Read the model definition and answer for the solid it produces. Units are mm, in the model's axes. A direction names the side the tool comes from. Give positions to 0.01 mm unless a question says otherwise; leave off trailing zeros. Write each loop counter-clockwise with the first axis right and the second up, starting at its lowest first coordinate (ties: lowest second). Pieces come first, ordered by that corner, then holes. Notation, with made-up numbers: M 77,-25.75 L 120,-25.75 A21 ccw 120,-4.75 Z; hole C 6,-2.5 d6. An arc over 180 degrees is marked long. Use a Markdown table: item, result. Add a question column.
Item 1: A cutting plane is placed at C-C on z = -16. Determine the outline of the cut face in (x, y), then the cut area to 3 significant figures.
Item 2: A cutting plane is placed at B-B on y = -10. Determine the outline of the cut face in (x, z), then the cut area to 3 significant figures.
Item 3: Given P1, Ø10, axis at x = 15, z = 5, coming from the +Y side; P2, Ø5, axis at x = 5, z = -15.5, coming from the -Y side; P3, Ø5, axis at x = -10.5, y = -17, coming from the -Z side, each flat-ended and moving along its own axis, determine where each tip first touches the part or whether it passes through.
Item 4: A cutting plane is placed at A-A on x = 0. Determine the outline of the cut face in (y, z), then the cut area to 3 significant figures.
Item 5: The mould has two halves that part along X. Classify faces 1 (the flat face through (25.588, -25, 0)), 2 (the cylindrical face through (-19.523, -50.493, 0.282)), 3 (the flat face through (-13, -51, 0)), 4 (the flat face through (-24.412, -25, 0)): pulls with the +X half, pulls with the -X half, needs draft (parallel to the pull), parting line crosses it, or undercut.
Item 6: For faces 5 (the flat face through (0, -25, 25.086)), 6 (the cylindrical face through (-0.98, -33.78, -25.41)), 7 (the flat face through (0, -50, 0)), determine the directions among +Z, -Z, +X, -X, +Y, -Y from which every point of the face is accessible in a straight line to the end or side of a thin tool.
Item 7: Consider probe 1 along Y at (x, z) = (-12, -8.5); probe 2 along Z at (x, y) = (-7, -20). Determine where each line is inside the solid, lowest interval first. Write a range as [from, to].
from build123d import *

# Parameters (mm, degrees)
F0_W     = 50
F0_H     = 50
F1_DEPTH = 50
F2_R     = 7.52824
F3_DEPTH = 1
F4_R     = 6.420566
F4_R_2   = 6.569333
F5_DEPTH = 1


with BuildPart() as f1:
    # F0 (on Front) → F1 (new body)
    with BuildSketch(Plane.XZ):
        with Locations((0.587589, 0.085707)):
            Rectangle(F0_W, F0_H)
    extrude(amount=F1_DEPTH)

    # F2 (on face) → F3 (join)
    with BuildSketch(Plane(origin=(0, 0, -24.914293), x_dir=(1, 0, 0), z_dir=(0, 0, -1))):
        with Locations((0, 26.31426)):
            Circle(F2_R)
    extrude(amount=F3_DEPTH)

    # F4 (on face) → F5 (join)
    with BuildSketch(Plane.XZ.offset(50)):
        with Locations((-13.108936, 0)):
            Circle(F4_R)
        with Locations((14.265605, 0)):
            Circle(F4_R_2)
    extrude(amount=F5_DEPTH)


solid = f1.part
Filled in:
| question | item | result |
|---|---|---|
| 1 | outline | M -24.41,-50 L 25.59,-50 L 25.59,0 L -24.41,0 Z |
| 1 | area | 2,500 mm² |
| 2 | outline | M -24.41,-24.91 L 25.59,-24.91 L 25.59,25.09 L -24.41,25.09 Z |
| 2 | area | 2,500 mm² |
| 3 | P1 | y = 0 |
| 3 | P2 | y = -50 |
| 3 | P3 | z = -24.91 |
| 4 | outline | M -50,-24.91 L -33.84,-24.91 L -33.84,-25.91 L -18.79,-25.91 L -18.79,-24.91 L 0,-24.91 L 0,25.09 L -50,25.09 Z |
| 4 | area | 2,520 mm² |
| 5 | face 1 | pulls with the +X half |
| 5 | face 2 | undercut |
| 5 | face 3 | needs draft |
| 5 | face 4 | pulls with the -X half |
| 6 | face 5 | +Z, +X, -X, +Y, -Y |
| 6 | face 6 | -Z |
| 6 | face 7 | -Y |
| 7 | probe 1 | [-50, 0] |
| 7 | probe 2 | [-24.91, 25.09] |
